Source: CAD feature listing. Evaluate the final solid. Frame: model axes, mm. A direction names the side the tool comes from. Give positions to 0.01 mm unless a question says otherwise; leave off trailing zeros. Write each loop counter-clockwise with the first axis right and the second up, starting at its lowest first coordinate (ties: lowest second). Pieces come first, ordered by that corner, then holes. Notation, with made-up numbers: (24, 75.25) - (51, 75.25) arc R18 cw to (51, 93.25) - close; hole circle Ø1 at (8.5, -29). An arc over 180 degrees is marked (long way). Answer as a JSON object with one key per item and string values. Group by question number.
from build123d import *

# Parameters (mm, degrees)
SKETCH1_W           = 117.4
SKETCH1_H           = 55.4
BOSS_EXTRUDE1_DEPTH = 1
SKETCH2_W           = 7
SKETCH2_H           = 7
BOSS_EXTRUDE2_DEPTH = 3
SKETCH3_R           = 1.35
CUT_EXTRUDE1_DEPTH  = 5
SKETCH7_W           = 30
SKETCH7_H           = 6
CUT_EXTRUDE5_DEPTH  = 5
SKETCH9_R           = 2.5
CUT_EXTRUDE6_DEPTH  = 3
SKETCH10_W          = 117.4
SKETCH10_H          = 1
BOSS_EXTRUDE3_DEPTH = 9


with BuildPart() as part:
    # Sketch1 → Boss-Extrude1 (new body)
    with BuildSketch(Plane(origin=(0, 0, 0), x_dir=(1, 0, 0), z_dir=(0, 1, 0))):
        Rectangle(SKETCH1_W, SKETCH1_H)
    extrude(amount=BOSS_EXTRUDE1_DEPTH)

    # Sketch2 → Boss-Extrude2 (add)
    with BuildSketch(Plane(origin=(0, 1, 0), x_dir=(1, 0, 0), z_dir=(0, 1, 0))):
        with Locations((55.2, 24.2)):
            Rectangle(SKETCH2_W, SKETCH2_H)
        with Locations((-55.2, 24.2)):
            Rectangle(SKETCH2_W, SKETCH2_H)
        with Locations((55.2, -24.2)):
            Rectangle(SKETCH2_W, SKETCH2_H)
        with Locations((-55.2, -24.2)):
            Rectangle(SKETCH2_W, SKETCH2_H)
    extrude(amount=BOSS_EXTRUDE2_DEPTH)

    # Sketch3 → Cut-Extrude1 (cut, through all)
    with BuildSketch(Plane(origin=(0, 4, 0), x_dir=(1, 0, 0), z_dir=(0, 1, 0))):
        with Locations((-55.5, 24.5)):
            Circle(SKETCH3_R)
        with Locations((55.5, 24.5)):
            Circle(SKETCH3_R)
        with Locations((55.5, -24.5)):
            Circle(SKETCH3_R)
        with Locations((-55.5, -24.5)):
            Circle(SKETCH3_R)
    extrude(amount=-CUT_EXTRUDE1_DEPTH, mode=Mode.SUBTRACT)

    # Sketch7 → Cut-Extrude5 (cut, through all)
    with BuildSketch(Plane.XZ):
        with Locations((36.7, 24.7)):
            Rectangle(SKETCH7_W, SKETCH7_H)
    extrude(amount=-CUT_EXTRUDE5_DEPTH, mode=Mode.SUBTRACT)

    # Sketch9 → Cut-Extrude6 (cut)
    with BuildSketch(Plane(origin=(0, 4, 0), x_dir=(1, 0, 0), z_dir=(0, 1, 0))):
        with Locations((-55.5, 24.5)):
            Circle(SKETCH9_R)
        with Locations((55.5, 24.5)):
            Circle(SKETCH9_R)
        with Locations((55.5, -24.5)):
            Circle(SKETCH9_R)
        with Locations((-55.5, -24.5)):
            Circle(SKETCH9_R)
    extrude(amount=-CUT_EXTRUDE6_DEPTH, mode=Mode.SUBTRACT)

    # Sketch10 → Boss-Extrude3 (add)
    with BuildSketch(Plane(origin=(0, 1, 0), x_dir=(1, 0, 0), z_dir=(0, 1, 0))):
        with Locations((0, -21.2)):
            Rectangle(SKETCH10_W, SKETCH10_H)
    extrude(amount=BOSS_EXTRUDE3_DEPTH)


solid = part.part
Q1. Reachability of faces 1 (the flat face through (-16, 1, 25)), 2 (the flat face through (52.8, 4, 24.7)), 3 (the flat face through (-55, 2, -20.7)), 4 (the flat face through (57, 1, 26)), 5 (the flat face through (-54, 4, -22)) from +Z, -Z, +X, -X, +Y, -Y: full face, straight path, thin tool, end or side. Return the list, or none.
Q2. Section B-B on y = 2.75. Return the cut outline in (x, z), then the cut area to 3 significant figures.
Q3. Section C-C on x = 55.5. Return the cut outline in (y, z).
Q4. Section A-A on z = 24.5. Return the cut outline in (x, y), then the cut area to 3 significant figures.
Q5. Section D-D on z = -24.5. Return the cut outline in (x, y), then the cut area to 3 significant figures.
Q6. Draft query along Z for faces 6 (the flat face through (-54, 1, 26)), 7 (the flat face through (-51.7, 2, -24)), 8 (the flat face through (-24.6, 0.5, 27.7)), 9 (the flat face through (55, 2, -20.7)). Return one class per face: released by +Z, released by -Z, zero draft, split by the parting line, or undercut.
Q7. Ray query, probe 1 along Z at (x, y) = (-55.5, 2.6); probe 2 along Z at (x, y) = (55.5, 0.6); probe 3 along X at (y, z) = (0.5, -24.5). Return the intervals inside material, ascending. Write a range as [from, to].
Q8. First-contact query: pin 1 Ø3 at (x, z) = (-3, 25.5) entering from +Y; pin 2 Ø5.5 at (x, z) = (56.5, 23.5) entering from +Y; pin 3 Ø1 at (x, y) = (-25.5, 8) entering from -Z; pin 4 Ø5.5 at (x, z) = (54, -25.5) entering from +Y. Flat tips, straight axial feed; report the tip coordinate or a pass-through.
Taken from the geometry:
{
 "1": {"face 1": "+Z, +Y", "face 2": "+Z, +X, -X, +Y", "face 3": "+X, -X, +Y", "face 4": "+Y", "face 5": "-Z, +X, -X, +Y"},
 "2": {"outline": "(-58.7, -27.7) - (-51.7, -27.7) - (-51.7, -20.7) - (-58.7, -20.7) - close; (-58.7, 20.7) - (58.7, 20.7) - (58.7, 27.7) - (51.7, 27.7) - (51.7, 21.7) - (-51.7, 21.7) - (-51.7, 27.7) - (-58.7, 27.7) - close; (51.7, -27.7) - (58.7, -27.7) - (58.7, -20.7) - (51.7, -20.7) - close; hole circle Ø5 at (-55.5, -24.5); hole circle Ø5 at (-55.5, 24.5); hole circle Ø5 at (55.5, -24.5); hole circle Ø5 at (55.5, 24.5)", "area": "221 mm²"},
 "3": {"outline": "(0, -27.7) - (4, -27.7) - (4, -27) - (1, -27) - (1, -25.85) - (0, -25.85) - close; (0, -23.15) - (1, -23.15) - (1, -22) - (4, -22) - (4, -20.7) - (1, -20.7) - (1, 20.7) - (10, 20.7) - (10, 21.7) - (4, 21.7) - (4, 22) - (1, 22) - (1, 23.15) - (0, 23.15) - close; (0, 25.85) - (1, 25.85) - (1, 27) - (4, 27) - (4, 27.7) - (0, 27.7) - close"},
 "4": {"outline": "(-58.7, 0) - (-56.85, 0) - (-56.85, 1) - (-58, 1) - (-58, 4) - (-58.7, 4) - close; (-54.15, 0) - (21.7, 0) - (21.7, 1) - (-51.7, 1) - (-51.7, 4) - (-53, 4) - (-53, 1) - (-54.15, 1) - close; (51.7, 0) - (54.15, 0) - (54.15, 1) - (53, 1) - (53, 4) - (51.7, 4) - close; (56.85, 0) - (58.7, 0) - (58.7, 4) - (58, 4) - (58, 1) - (56.85, 1) - close", "area": "94.0 mm²"},
 "5": {"outline": "(-58.7, 0) - (-56.85, 0) - (-56.85, 1) - (-58, 1) - (-58, 4) - (-58.7, 4) - close; (-54.15, 0) - (54.15, 0) - (54.15, 1) - (53, 1) - (53, 4) - (51.7, 4) - (51.7, 1) - (-51.7, 1) - (-51.7, 4) - (-53, 4) - (-53, 1) - (-54.15, 1) - close; (56.85, 0) - (58.7, 0) - (58.7, 4) - (58, 4) - (58, 1) - (56.85, 1) - close", "area": "124 mm²"},
 "6": {"face 6": "undercut", "face 7": "zero draft", "face 8": "released by +Z", "face 9": "undercut"},
 "7": {"probe 1": "z = [-27.7, -27], [-22, -20.7], [20.7, 22], [27, 27.7]", "probe 2": "z = [-27.7, -25.85], [-23.15, 23.15], [25.85, 27.7]", "probe 3": "x = [-58.7, -56.85], [-54.15, 54.15], [56.85, 58.7]"},
 "8": {"pin 1": "stops at y = 1", "pin 2": "stops at y = 10", "pin 3": "stops at z = 20.7", "pin 4": "stops at y = 4"}
}
